For this review, take the finished solid that the model builds, in its own axes (mm). Give positions to 0.01 mm unless a question says otherwise; leave off trailing zeros. Order: outer loops, then holes, each group sorted by start corner. A loop starts at its lowest first (then second) coordinate and runs counter-clockwise, first axis right, second up. Notation, with made-up numbers: (59.5, 51.25) - (81.5, 51.25) arc R26 cw to (81.5, 74.25) - close; hole circle Ø7 at (78, 26). An arc over 180 degrees is marked (long way). One line per item, written item: value.
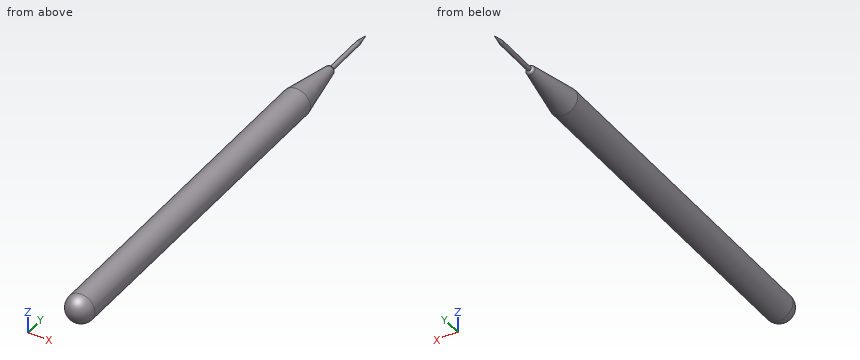
```python
from build123d import *

# Parameters (mm, degrees)
SKETCH1_R           = 5
BOSS_EXTRUDE1_DEPTH = 75
CHAMFER1_SIZE       = 20
CHAMFER1_SIZE2      = 3.526539614
FILLET1_R           = 5
SKETCH2_R           = 0.75
BOSS_EXTRUDE2_DEPTH = 20
CHAMFER2_SIZE       = 4
CHAMFER2_SIZE2      = 0.705307923
FILLET2_R           = 1


with BuildPart() as part:
    # Sketch1 → Boss-Extrude1 (new, symmetric)
    with BuildSketch(Plane(origin=(0, 0, 0), x_dir=(1, 0, 0), z_dir=(0, 1, 0))):
        with Locations(Location((0, 0, 0), (0, 0, 270))):
            Circle(SKETCH1_R)
    extrude(amount=BOSS_EXTRUDE1_DEPTH, both=True)

    # Chamfer1
    chamfer1_edges = [part.edges().sort_by_distance(p)[0] for p in [
        (0, 75, -5),
    ]]
    chamfer1_side = [part.faces().sort_by_distance(p)[0] for p in [
        (0, 0, -5),
    ]]
    chamfer(chamfer1_edges, length=CHAMFER1_SIZE, length2=CHAMFER1_SIZE2, reference=chamfer1_side[0])

    # Fillet1
    fillet1_edges = [part.edges().sort_by_distance(p)[0] for p in [
        (0, -75, -5),
    ]]
    fillet(fillet1_edges, radius=FILLET1_R)

    # Sketch2 → Boss-Extrude2 (add)
    with BuildSketch(Plane(origin=(0, 75, 0), x_dir=(1, 0, 0), z_dir=(0, 1, 0))):
        with Locations(Location((0, 0, 0), (0, 0, 270))):
            Circle(SKETCH2_R)
    extrude(amount=BOSS_EXTRUDE2_DEPTH)

    # Chamfer2
    chamfer2_edges = [part.edges().sort_by_distance(p)[0] for p in [
        (0, 95, -0.75),
    ]]
    chamfer2_side = [part.faces().sort_by_distance(p)[0] for p in [
        (0, 85, -0.75),
    ]]
    chamfer(chamfer2_edges, length=CHAMFER2_SIZE, length2=CHAMFER2_SIZE2, reference=chamfer2_side[0])

    # Fillet2
    # the kernel refuses this fillet: 1 mm, written as the material it takes off along each edge
    with BuildSketch(Plane(origin=(0, 75, 0), x_dir=(0, 0, 1), z_dir=(-1, 0, 0))) as fillet2_piece_1:
        with BuildLine():
            CenterArc((0.6331529, -0.993149916), FILLET2_R, 10, 73.289825559)
            Line((1.617960653, -0.819501738), (1.637656808, -0.816028775))
            Line((1.637656808, -0.816028775), (1.493156541, 0.003472964))
            Line((1.493156541, 0.003472964), (1.473460386, 0.02))
            ThreePointArc((1.473460386, 0.02), (1.111730193, 0.02), (0.752336942, 0.019862998))
            Line((0.752336942, 0.019862998), (0.75, 0))
        make_face()
    revolve(axis=Axis((0, 75, 0), (0, 1, 0)), mode=Mode.SUBTRACT)


solid = part.part
```
(1) Take a section at A-A (y = -47.5). Write out the cut boundary in (x, z), then the cut area to 3 significant figures.
Answers below:
outline: circle Ø10 at (0, 0)
area: 78.5 mm^2
(2) For P1, Ø1, axis at y = 49.5, z = -2, coming from the +X side; P2, Ø6, axis at x = 1, y = 65, coming from the -Z side, all flat-tipped, find the tip position at first contact; note any pin that passes through.
Answers below:
P1: stops at x = 4.77
P2: stops at z = -3.74
(3) Take a section at B-B (y = 57). Write out the cut boundary in (x, z).
Answers below:
outline: circle Ø9.29 at (0, 0)
(4) Wall thickness on line 1 (X direction, y = -67.5, z = -0.5); line 2 (X direction, y = 24, z = -4.25); line 3 (Z direction, x = -3.5, y = -39): over which ranges is each line inside the solid? List them lowest first. Write a range as from..to.
Answers below:
line 1: x = -4.97..4.97
line 2: x = -2.63..2.63
line 3: z = -3.57..3.57
